CAD build for the part. Positions are in the model's coordinates, mm. A direction names the side the tool comes from. Give positions to 0.01 mm unless a question says otherwise; leave off trailing zeros. Loops run counter-clockwise (first coordinate to the right, second up) from the corner with the lowest first, then second, coordinate; pieces in that order, holes last. Notation, with made-up numbers: M 18.25,18 L 68.25,18 A10 cw 68.25,29 Z; hole C 10,59.25 d5. An arc over 180 degrees is marked long. Answer as CSV lines item,"result".
```python
from build123d import *

# Parameters (mm, degrees)
F0_R     = 31.5
F0_R_2   = 26.9875
F1_DEPTH = 45
F0_R_3   = 39.5
F0_R_4   = 2
F2_DEPTH = 16
F0_R_5   = 2.5
F0_R_6   = 4
F3_DEPTH = 49.5


with BuildPart() as f1:
    # F0 (on Right) → F1 (new body)
    with BuildSketch(Plane.YZ):
        Circle(F0_R)
        Circle(F0_R_2, mode=Mode.SUBTRACT)
    extrude(amount=F1_DEPTH)

    # F0 (on Right) → F2 (join)
    with BuildSketch(Plane.YZ):
        Circle(F0_R_3)
        with Locations((-25.090836, -25.090836)):
            Circle(F0_R_4, mode=Mode.SUBTRACT)
        with Locations((0, -35.4838)):
            Circle(F0_R_4, mode=Mode.SUBTRACT)
        with Locations((25.090836, -25.090836)):
            Circle(F0_R_4, mode=Mode.SUBTRACT)
        with Locations((-35.4838, 0)):
            Circle(F0_R_4, mode=Mode.SUBTRACT)
        with Locations((-25.090836, 25.090836)):
            Circle(F0_R_4, mode=Mode.SUBTRACT)
        Circle(F0_R, mode=Mode.SUBTRACT)
        with Locations((35.4838, 0)):
            Circle(F0_R_4, mode=Mode.SUBTRACT)
        with Locations((0, 35.4838)):
            Circle(F0_R_4, mode=Mode.SUBTRACT)
        with Locations((25.090836, 25.090836)):
            Circle(F0_R_4, mode=Mode.SUBTRACT)
    extrude(amount=F2_DEPTH)

    # F0 (on Right) → F3 (join)
    with BuildSketch(Plane.YZ):
        Circle(F0_R_2)
        with Locations((-17.102703, -9.87425)):
            Circle(F0_R_5, mode=Mode.SUBTRACT)
        with Locations((0, -19.7485)):
            Circle(F0_R_5, mode=Mode.SUBTRACT)
        with Locations((17.102703, -9.87425)):
            Circle(F0_R_5, mode=Mode.SUBTRACT)
        with Locations((-17.102703, 9.87425)):
            Circle(F0_R_5, mode=Mode.SUBTRACT)
        Circle(F0_R_6, mode=Mode.SUBTRACT)
        with Locations((17.102703, 9.87425)):
            Circle(F0_R_5, mode=Mode.SUBTRACT)
        with Locations((0, 19.7485)):
            Circle(F0_R_5, mode=Mode.SUBTRACT)
    extrude(amount=F3_DEPTH)


solid = f1.part
```
Q1. Wall check: line 1 (X direction, y = -28.5, z = -9.5); line 2 (X direction, y = 11.5, z = -32.5); line 3 (Y direction, x = 36, z = -12). Give the ranges that are in metal, low to high. Write a range as [from, to].
Solution:
line 1,"x = [0, 45]"
line 2,"x = [0, 16]"
line 3,"y = [-29.12, -18.42], [-15.79, 15.79], [18.42, 29.12]"
Q2. Cut at A-A (z = 0). Write the cut outline in (x, y), and give its area (3 significant figures).
Solution:
outline,"M 0,-39.5 L 16,-39.5 L 16,-37.48 L 0,-37.48 Z; M 0,-33.48 L 16,-33.48 L 16,-31.5 L 45,-31.5 L 45,-26.99 L 49.5,-26.99 L 49.5,-4 L 0,-4 Z; M 0,4 L 49.5,4 L 49.5,26.99 L 45,26.99 L 45,31.5 L 16,31.5 L 16,33.48 L 0,33.48 Z; M 0,37.48 L 16,37.48 L 16,39.5 L 0,39.5 Z"
area,"2,810 mm²"
Q3. Which spindle directions (+Z, -Z, +X, -X, +Y, -Y) get a long thin tool onto all of the face, cutting with end or side? Do faces 4 (the cylindrical face through (7.888, 24.83, 27.074)), 5 (the cylindrical face through (30.297, -4.101, 31.232)). Say none if no direction does.
Solution:
face 4,"+X, -X"
face 5,"+X"
Q4. Cut at C-C (y = 0). Give the number of separate pieces and of enclosed holes in the cut face, and give its area (3 significant figures).
Solution:
separate pieces,"6"
enclosed holes,"0"
area,"2,310 mm²"
Q5. Mould opens along Y. For faces 1 (the cylindrical face through (7.89, -33.64, -0.77)), 2 (the flat face through (49.5, 6, 0)), 3 (the cylindrical face through (7.89, -29.11, 26.7)) say: released by +Y, released by -Y, zero draft, split by the parting line, or undercut.
Solution:
face 1,"undercut"
face 2,"zero draft"
face 3,"split by the parting line"
Q6. Pin check, flat tips, straight feed: P1, Ø12, axis at y = 21.5, z = 30.5, coming from the +X side; P2, Ø12, axis at y = 13.5, z = 10.5, coming from the -X side; P3, Ø12, axis at x = 33.5, y = -28, coming from the +Z side; P4, Ø12, axis at x = 18.5, z = 27.5, coming from the -Y side. Stop position of each tip, or through.
Solution:
P1,"stops at x = 45"
P2,"stops at x = 0"
P3,"stops at z = 22.54"
P4,"stops at y = -32.78"
Q7. Cut at B-B (y = 17). Write the cut outline in (x, z), and give its area (3 significant figures).
Solution:
outline,"M 0,-35.65 L 16,-35.65 L 16,-26.52 L 45,-26.52 L 45,-20.96 L 49.5,-20.96 L 49.5,-12.37 L 0,-12.37 Z; M 0,-7.38 L 49.5,-7.38 L 49.5,7.38 L 0,7.38 Z; M 0,12.37 L 49.5,12.37 L 49.5,20.96 L 45,20.96 L 45,26.52 L 16,26.52 L 16,35.65 L 0,35.65 Z"
area,"2,370 mm²"
